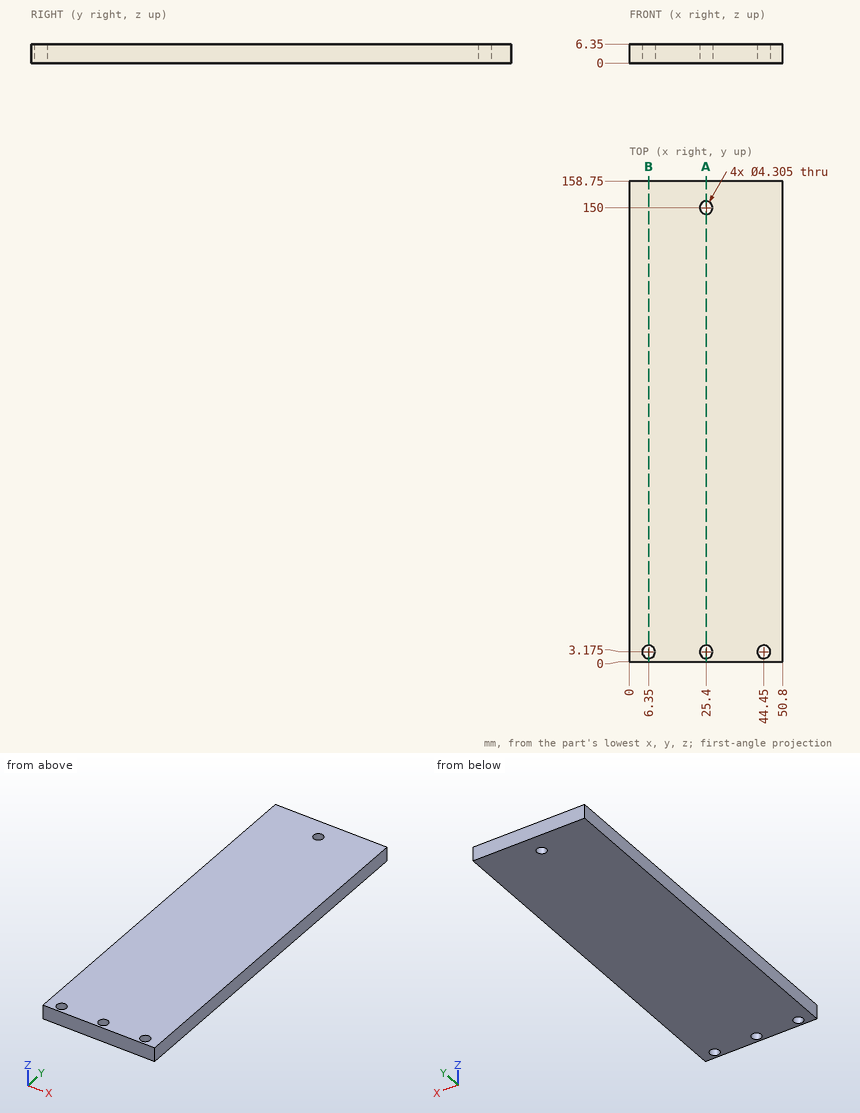
Design review of the part shown in the three views and the two pictorial views. Dimensions are in mm from the part's minimum x, y and z. Coordinates: 2 decimals unless noted, no trailing zeros. Order: outer loops, then holes, each group sorted by start corner. A loop starts at its lowest first (then second) coordinate and runs counter-clockwise, first axis right, second up. Notation, with made-up numbers: (73.25, 51.25) - (111.25, 51.25) arc R31 ccw to (111.25, 75.25) - close; hole circle Ø11 at (-39.75, -33). An arc over 180 degrees is marked (long way). One line per question, with ' | ' between items.
Q1. Consider section B-B, the plane x = 6.35. Give the boundary of the cut face in (y, z), then the cut area to 3 significant figures.
Answer key:
outline: (0, 0) - (1.02, 0) - (1.02, 6.35) - (0, 6.35) - close; (5.33, 0) - (158.75, 0) - (158.75, 6.35) - (5.33, 6.35) - close | area: 981 mm2
Q2. Clearance check with flat-ended pins moving along their axes: pin 1 Ø3.5 at (x, y) = (44.45, 3.175) entering from -Z; pin 2 Ø5.5 at (x, y) = (25.4, 150) entering from +Z. State where each tip first meets the part, or that it passes through.
Answer key:
pin 1: passes through | pin 2: stops at z = 6.35
Q3. Consider section A-A, the plane x = 25.4. Give the boundary of the cut face in (y, z).
Answer key:
outline: (0, 0) - (1.02, 0) - (1.02, 6.35) - (0, 6.35) - close; (5.33, 0) - (147.85, 0) - (147.85, 6.35) - (5.33, 6.35) - close; (152.15, 0) - (158.75, 0) - (158.75, 6.35) - (152.15, 6.35) - close
Q4. To check wall thickness, follow line 1 along Y through (x, z) = (6.35, 2.75); line 2 along Y through (x, z) = (45, 3.75). State the ranges of each line that lie inside material, in increasing order.
Answer key:
line 1: y = 0 to 1.02, 5.33 to 158.75 | line 2: y = 0 to 1.09, 5.26 to 158.75
